Geometry: final body of the model. Coordinates: model frame, mm. A direction names the side the tool comes from. Give positions to 0.01 mm unless a question says otherwise; leave off trailing zeros. Order: outer loops, then holes, each group sorted by start corner. A loop starts at its lowest first (then second) coordinate and runs counter-clockwise, first axis right, second up. Notation, with made-up numbers: (28, 82) -> (79, 82) arc R14 cw to (79, 106) -> close; hole circle Ø9 at (-19, 38.25). An arc over 180 degrees is marked (long way). Write item = value, one per line.
```python
from build123d import *

# Parameters (mm, degrees)
CYLINDER001_R               = 2.1
CYLINDER001_DEPTH           = 10
CYLINDER001_PLACEMENT_ANGLE = 45
CYLINDER_R                  = 2.1
CYLINDER_DEPTH              = 10
PAD_DEPTH                   = 10


with BuildPart() as insert_hole001:
    # Cylinder001 → Cylinder001 (new body)
    with BuildSketch(Plane.XY):
        Circle(CYLINDER001_R)
    extrude(amount=CYLINDER001_DEPTH)


with BuildPart() as insert_hole001_1:
    # Cylinder001 placement: moved
    add(insert_hole001.part.moved(Location((15.585786, 5, 9.899495))).rotate(Axis((15.585786, 5, 9.899495), (0, -1, 0)), CYLINDER001_PLACEMENT_ANGLE))


with BuildPart() as hole_fusion:
    # Cylinder → Cylinder (new body)
    with BuildSketch(Plane(origin=(17, 5, 0), x_dir=(1, 0, 0), z_dir=(0, 0, 1))):
        Circle(CYLINDER_R)
    extrude(amount=CYLINDER_DEPTH)

    # Fusion: union insert hole001
    add(insert_hole001_1.part)


with BuildPart() as angle_cut:
    # Sketch → Pad (new body)
    with BuildSketch(Plane.XZ):
        with BuildLine():
            Line((12.855752, 18.320889), (0, 3))
            ThreePointArc((0, 3), (-1.5, 1.5), (0, 0))
            Line((0, 0), (20, 0))
            ThreePointArc((20, 0), (21.5, 1.5), (20, 3))
            Line((20, 3), (3.916222, 3))
            Line((3.916222, 3), (15.153886, 16.392526))
            ThreePointArc((15.153886, 16.392526), (14.969, 18.505774), (12.855752, 18.320889))
        make_face()
    extrude(amount=-PAD_DEPTH)

    # Cut: cut hole fusion
    add(hole_fusion.part, mode=Mode.SUBTRACT)


solid = angle_cut.part
```
1) Section query A-A (x = 17). Output: boundary loops of the cut face in (y, z), plus the area to 3 significant figures.
Check sheet entries:
outline = (0, 0) -> (2.9, 0) -> (2.9, 3) -> (0, 3) -> close; (7.1, 0) -> (10, 0) -> (10, 3) -> (7.1, 3) -> close
area = 17.4 mm²
2) Section query D-D (y = 6.5). Output: boundary loops of the cut face in (x, z).
Check sheet entries:
outline = (0, 0) -> (15.53, 0) -> (15.53, 3) -> (3.92, 3) -> (11.44, 11.97) -> (9.31, 14.1) -> (0, 3) arc R1.5 ccw to start; (11.21, 16.36) -> (13.34, 14.23) -> (15.15, 16.39) arc R1.5 ccw to (12.86, 18.32) -> close; (18.47, 0) -> (20, 0) arc R1.5 ccw to (20, 3) -> (18.47, 3) -> close
3) Mould query, pull axis Z, two halves, no side actions, for faces 3 (the face through (10, 5, 0)), 4 (the face through (19.003, 5.631, 1.479)), 5 (the face through (21.5, 4.9, 1.5)), 6 (the face through (12, 5, 3)). Classes: +Z half, -Z half, draft (parallel to the pull), parting line (faces both ways), or undercut.
Check sheet entries:
face_3 = -Z half
face_4 = draft
face_5 = parting line
face_6 = undercut
4) Line query: line 1 (Y direction, x = 17, z = 2.2); line 2 (X direction, y = 5, z = 0.85); line 3 (X direction, y = 5, z = 1.65). Output: solid intervals per line, ascending. Write a range as from..to.
Check sheet entries:
line_1 = 0..2.9, 7.1..10
line_2 = -1.35..14.9, 19.1..21.35
line_3 = -1.49..14.9, 19.1..21.49
5) Section query B-B (y = 9). Output: boundary loops of the cut face in (x, z).
Check sheet entries:
outline = (0, 0) -> (20, 0) arc R1.5 ccw to (20, 3) -> (3.92, 3) -> (15.15, 16.39) arc R1.5 ccw to (12.86, 18.32) -> (0, 3) arc R1.5 ccw to start
6) First-contact query: P1, Ø1, axis at y = 3, z = 6.5, coming from the -X side; P2, Ø3.5, axis at x = 17, y = 5, coming from the +Z side; P3, Ø3, axis at x = 7.5, z = 17, coming from the +Y side. Flat tips, straight axial feed; report the tip coordinate or a pass-through.
Check sheet entries:
P1 = 2.52
P2 = 18.19
P3 = through
7) Section query C-C (z = 1.5). Output: boundary loops of the cut face in (x, y), plus the area to 3 significant figures.
Check sheet entries:
outline = (-1.5, 0) -> (21.5, 0) -> (21.5, 10) -> (-1.5, 10) -> close; hole circle Ø4.2 at (17, 5)
area = 216 mm²
8) Reachability of faces 1 (the face through (9.456, 4.93, 9.603)), 2 (the face through (14.994, 4.93, 18.484)) from +Z, -Z, +X, -X, +Y, -Y: full face, straight path, thin tool, end or side. Return the list, or none.
Check sheet entries:
face_1 = +X, +Y, -Y
face_2 = +Y, -Y
